from build123d import *

# Parameters (mm, degrees)
SKETCH_1_R          = 10
SKETCH_1_R_2        = 1.5
EXTRUDE_1_DEPTH     = 2.5
SKETCH_2_R          = 4.4
SKETCH_2_R_2        = 2.55
EXTRUDE_2_DEPTH     = 2
FILLET_1_R          = 0.5
CUT_EXTRUDE_START   = -1
SKETCH_3_R          = 2.55
CUT_EXTRUDE_1_DEPTH = 1


with BuildPart() as part:
    # 草图1 → 凸台-拉伸1 (new body)
    with BuildSketch(Plane(origin=(0, 0, 0), x_dir=(1, 0, 0), z_dir=(0, 1, 0))):
        with Locations(Location((0, 0, 0), (0, 0, 270))):
            Circle(SKETCH_1_R)
        with Locations(Location((7, 0, 0), (0, 0, 270))):
            Circle(SKETCH_1_R_2, mode=Mode.SUBTRACT)
        with Locations(Location((0, 7, 0), (0, 0, 270))):
            Circle(SKETCH_1_R_2, mode=Mode.SUBTRACT)
        with Locations(Location((0, -7, 0), (0, 0, 270))):
            Circle(SKETCH_1_R_2, mode=Mode.SUBTRACT)
        with Locations(Location((-7, 0, 0), (0, 0, 270))):
            Circle(SKETCH_1_R_2, mode=Mode.SUBTRACT)
        with Locations(Location((0, 0, 0), (0, 0, 270))):
            Circle(SKETCH_1_R_2, mode=Mode.SUBTRACT)
    extrude(amount=EXTRUDE_1_DEPTH)

    # 草图2 → 凸台-拉伸2 (add)
    with BuildSketch(Plane(origin=(0, 2.5, 0), x_dir=(1, 0, 0), z_dir=(0, 1, 0))):
        with Locations(Location((0, 0, 0), (0, 0, 270))):
            Circle(SKETCH_2_R)
        with Locations(Location((0, 0, 0), (0, 0, 270))):
            Circle(SKETCH_2_R_2, mode=Mode.SUBTRACT)
    extrude(amount=EXTRUDE_2_DEPTH)

    # 圆角1
    fillet_1_edges = [part.edges().sort_by_distance(p)[0] for p in [
        (0, 2.5, -4.4),
    ]]
    fillet(fillet_1_edges, radius=FILLET_1_R)

    # 草图3 → 切除-拉伸1 (cut)
    with BuildSketch(Plane(origin=(0, 2.5, 0), x_dir=(1, 0, 0), z_dir=(0, 1, 0)).offset(CUT_EXTRUDE_START)):
        with Locations(Location((0, 0, 0), (0, 0, 270))):
            Circle(SKETCH_3_R)
    extrude(amount=CUT_EXTRUDE_1_DEPTH, mode=Mode.SUBTRACT)


solid = part.part
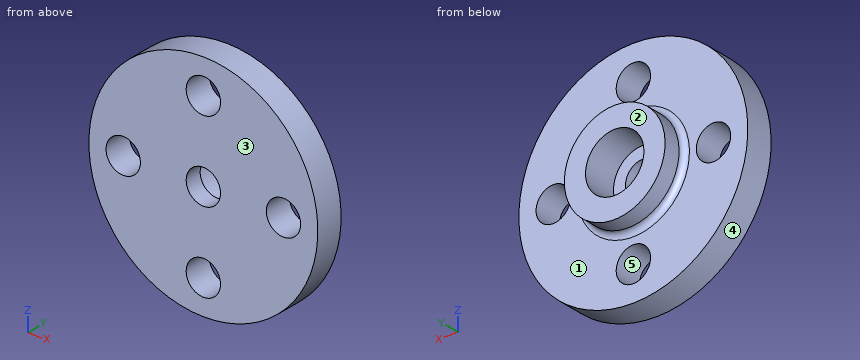
Geometry: final body of the model. Coordinates: model frame, mm. Face numbers are marked on the shaded views. A direction names the side the tool comes from. Give positions to 0.01 mm unless a question says otherwise; leave off trailing zeros. Loops run counter-clockwise (first coordinate to the right, second up) from the corner with the lowest first, then second, coordinate; pieces in that order, holes last. Notation, with made-up numbers: M 18,70.5 L 40,70.5 A24 ccw 40,90.5 Z; hole C 4,32.5 d9. An arc over 180 degrees is marked long. Put each result on its own line as item: value.
1) Cut plane C-C, the plane y = 0.9. Return the cut outline in (x, z).
Computed values:
outline: C 0,0 d20; hole C -7,0 d3; hole C 0,-7 d3; hole C 0,0 d3; hole C 0,7 d3; hole C 7,0 d3
2) Material intervals for L1, parallel to Z at x = -0.75, y = 2.45; L2, parallel to Y at x = 3.25, z = -6.25; L3, parallel to X at y = 2, z = -8, sorted ascending. Write a range as from..to.
Computed values:
L1: z = -9.97..-8.3, -5.7..-2.44, 2.44..5.7, 8.3..9.97
L2: y = 0..2.5
L3: x = -6..-1.12, 1.12..6
3) Reachability of the marked faces 1 and 2 from +Z, -Z, +X, -X, +Y, -Y: full face, straight path, thin tool, end or side. Return the list, or none.
Computed values:
face 1: +Y
face 2: +Z, -Z, +X, -X, +Y
4) Cut plane B-B, the plane x = 0. Return the cut outline in (y, z).
Computed values:
outline: M 0,-10 L 2.5,-10 L 2.5,-8.5 L 0,-8.5 Z; M 0,-5.5 L 2.5,-5.5 L 2.5,-4.9 A0.5 cw 3,-4.4 L 4.5,-4.4 L 4.5,-2.55 L 1.5,-2.55 L 1.5,-1.5 L 0,-1.5 Z; M 0,1.5 L 1.5,1.5 L 1.5,2.55 L 4.5,2.55 L 4.5,4.4 L 3,4.4 A0.5 cw 2.5,4.9 L 2.5,5.5 L 0,5.5 Z; M 0,8.5 L 2.5,8.5 L 2.5,10 L 0,10 Z
5) Mould query, pull axis X, two halves, no side actions, for the marked faces 3, 4 and 5. Classes: released by +X, released by -X, zero draft, split by the parting line, or undercut.
Computed values:
face 3: zero draft
face 4: split by the parting line
face 5: undercut
6) Cut plane A-A, the plane z = 0. Return the cut outline in (x, y).
Computed values:
outline: M -10,0 L -8.5,0 L -8.5,2.5 L -10,2.5 Z; M -5.5,0 L -1.5,0 L -1.5,1.5 L -2.55,1.5 L -2.55,4.5 L -4.4,4.5 L -4.4,3 A0.5 cw -4.9,2.5 L -5.5,2.5 Z; M 1.5,0 L 5.5,0 L 5.5,2.5 L 4.9,2.5 A0.5 cw 4.4,3 L 4.4,4.5 L 2.55,4.5 L 2.55,1.5 L 1.5,1.5 Z; M 8.5,0 L 10,0 L 10,2.5 L 8.5,2.5 Z
7) Cut plane D-D, the plane z = 7. Return the cut outline in (x, y).
Computed values:
outline: M -7.14,0 L -1.5,0 L -1.5,2.5 L -7.14,2.5 Z; M 1.5,0 L 7.14,0 L 7.14,2.5 L 1.5,2.5 Z
8) First-contact query: P1, Ø1, axis at y = 3.5, z = -2, coming from the -X side; P2, Ø3.5, axis at x = 0, z = -7, coming from the +Y side; P3, Ø4.5, axis at x = 0, z = 0, coming from the +Y side. Flat tips, straight axial feed; report the tip coordinate or a pass-through.
Computed values:
P1: stops at x = -4.14
P2: stops at y = 2.5
P3: stops at y = 1.5
